The listing builds one solid part. Answer for the finished solid, in the listing's coordinates (mm). Round coordinates to 2 decimals unless told otherwise and drop trailing zeros. Loops run counter-clockwise (first coordinate to the right, second up) from the corner with the lowest first, then second, coordinate; pieces in that order, holes last. Notation, with made-up numbers: (-24, 34) -> (-6, 34) arc R15 ccw to (-6, 38) -> close; hole circle Ø6 at (40, 77). An arc over 180 degrees is marked (long way). Use a Markdown table: item, result. Add a question column.
Q1. Consider line 1 (Z direction, x = -1, y = 4); line 2 (X direction, y = 4.35, z = -15); line 3 (Y direction, x = 0.25, z = 2.25). Determine where each line is inside the solid, lowest interval first.
Q2. For a pull along Z with two mould halves and no side action, classify faces 1 (the cylindrical face through (-0.97, 2.96, -1.27)), 2 (the cylindrical face through (-3.2, 5.7, -4.25)), 3 (the flat face through (-9, 0, -5)), 4 (the cylindrical face through (-14, 2.96, -16.18)) as released by +Z, released by -Z, zero draft, split by the parting line, or undercut.
Q3. Section A-A on y = 2.75 is taken. Give the vertices of the cut face in (x, z).
Q4. Given pin 1 Ø1.5 at (x, z) = (-10, -13) entering from +Y; pin 2 Ø1 at (x, y) = (-14.5, 4.5) entering from +Z, each flat-ended and moving along its own axis, determine where each tip first touches the part or whether it passes through.
from build123d import *

# Parameters (mm, degrees)
SKETCH1_R           = 1.6
BOSS_EXTRUDE1_DEPTH = 6
FILLET2_R           = 1


with BuildPart() as part:
    # Sketch1 → Boss-Extrude1 (new body)
    with BuildSketch(Plane(origin=(0, 0, 0), x_dir=(1, 0, 0), z_dir=(0, 1, 0))):
        with BuildLine():
            Line((-17.848575481, 13.84458241), (-13.415177199, 3.22141215))
            ThreePointArc((-13.415177199, 3.22141215), (-12.76227277, 2.249875109), (-11.787276601, 1.60214763))
            Line((-11.787276601, 1.60214763), (-1.140674884, -2.77468211))
            ThreePointArc((-1.140674884, -2.77468211), (2.77468211, -1.140674884), (1.140674884, 2.77468211))
            Line((1.140674884, 2.77468211), (-7.207304912, 6.206545835))
            ThreePointArc((-7.207304912, 6.206545835), (-8.18230108, 6.854273314), (-8.835205509, 7.825810355))
            Line((-8.835205509, 7.825810355), (-12.311424519, 16.15541759))
            ThreePointArc((-12.311424519, 16.15541759), (-16.23541759, 17.768575481), (-17.848575481, 13.84458241))
        make_face()
        with Locations(Location((-15.08, 15, 0), (0, 0, 270))):
            Circle(SKETCH1_R, mode=Mode.SUBTRACT)
        with Locations(Location((0, 0, 0), (0, 0, 270))):
            Circle(SKETCH1_R, mode=Mode.SUBTRACT)
    extrude(amount=BOSS_EXTRUDE1_DEPTH)

    # Fillet2
    fillet2_edges = [part.edges().sort_by_distance(p)[0] for p in [
        (-15.63187634, 0, -8.53299728),
        (-16.23541759, 0, -17.768575481),
        (-10.573315014, 0, -11.990613972),
        (-8.18230108, 0, -6.854273314),
        (-16.23541759, 6, -17.768575481),
        (-15.63187634, 6, -8.53299728),
        (-12.76227277, 6, -2.249875109),
        (-6.463975743, 6, 0.58626724),
        (2.77468211, 6, 1.140674884),
        (-3.033315014, 6, -4.490613972),
        (-8.18230108, 6, -6.854273314),
        (-3.033315014, 0, -4.490613972),
        (-10.573315014, 6, -11.990613972),
        (2.77468211, 0, 1.140674884),
        (-6.463975743, 0, 0.58626724),
        (-12.76227277, 0, -2.249875109),
    ]]
    fillet(fillet2_edges, radius=FILLET2_R)


solid = part.part
Checked values:
| question | item | result |
|---|---|---|
| 1 | line 1 | z = -3.65 to -1.25, 1.25 to 2.83 |
| 1 | line 2 | x = -18.08 to -16.68, -13.48 to -11.83 |
| 1 | line 3 | y = 0.04 to 5.96 |
| 2 | face 1 | undercut |
| 2 | face 2 | released by -Z |
| 2 | face 3 | zero draft |
| 2 | face 4 | undercut |
| 3 | outline | (-17.85, -13.84) arc R3 ccw to (-12.31, -16.16) -> (-8.84, -7.83) arc R3 cw to (-7.21, -6.21) -> (1.14, -2.77) arc R3 ccw to (-1.14, 2.77) -> (-11.79, -1.6) arc R3 ccw to (-13.42, -3.22) -> close; hole circle Ø3.2 at (-15.08, -15); hole circle Ø3.2 at (0, 0) |
| 4 | pin 1 | passes through |
| 4 | pin 2 | stops at z = -4.62 |
